```python
from build123d import *

# Parameters (mm, degrees)
SKETCH_1_W          = 30
SKETCH_1_H          = 20
EXTRUDE_1_DEPTH     = 30
SKETCH_3_W          = 25
SKETCH_3_H          = 16.07
EXTRUDE_2_DEPTH     = 10
SKETCH_7_W          = 8
SKETCH_7_H          = 10.5
CUT_EXTRUDE_1_DEPTH = 45.426074479
SKETCH_9_W          = 17
SKETCH_9_H          = 26
CUT_EXTRUDE_2_DEPTH = 25
SKETCH_11_R         = 1.4
EXTRUDE_3_DEPTH     = 4
SKETCH_12_R         = 1.4
EXTRUDE_4_DEPTH     = 4


with BuildPart() as part:
    # 草图1 → 凸台-拉伸1 (new body)
    with BuildSketch(Plane(origin=(0, 0, 0), x_dir=(1, 0, 0), z_dir=(0, 1, 0))):
        with Locations((-0.371492922, 2.183544304)):
            Rectangle(SKETCH_1_W, SKETCH_1_H)
    extrude(amount=EXTRUDE_1_DEPTH)

    # 草图3 → 凸台-拉伸2 (add)
    with BuildSketch(Plane.XY.offset(7.816455696)):
        with Locations((-0.371492922, 15)):
            Rectangle(SKETCH_3_W, SKETCH_3_H)
    extrude(amount=EXTRUDE_2_DEPTH)

    # 草图7 → 切除-拉伸1 (cut, through all)
    with BuildSketch(Plane.ZY.offset(12.871492922)):
        with Locations((13.816455696, 15)):
            Rectangle(SKETCH_7_W, SKETCH_7_H)
    extrude(amount=-CUT_EXTRUDE_1_DEPTH, mode=Mode.SUBTRACT)

    # 草图9 → 切除-拉伸2 (cut)
    with BuildSketch(Plane.ZY.offset(15.371492922)):
        with Locations((-2.183544304, 15)):
            Rectangle(SKETCH_9_W, SKETCH_9_H)
    extrude(amount=-CUT_EXTRUDE_2_DEPTH, mode=Mode.SUBTRACT)

    # 草图11 → 凸台-拉伸3 (add)
    with BuildSketch(Plane(origin=(14.628507078, 0, 0), x_dir=(0, 0, -1), z_dir=(1, 0, 0))):
        with Locations(Location((-2.116455696, 7, 0), (0, 0, 180))):
            Circle(SKETCH_11_R)
        with Locations(Location((6.483544304, 7, 0), (0, 0, 180))):
            Circle(SKETCH_11_R)
    extrude(amount=EXTRUDE_3_DEPTH)

    # 草图12 → 凸台-拉伸4 (add)
    with BuildSketch(Plane(origin=(0, 0, -12.183544304), x_dir=(-1, 0, 0), z_dir=(0, 0, -1))):
        with Locations(Location((-3.928507078, 7, 0), (0, 0, 180))):
            Circle(SKETCH_12_R)
        with Locations(Location((4.671492922, 7, 0), (0, 0, 180))):
            Circle(SKETCH_12_R)
    extrude(amount=EXTRUDE_4_DEPTH)


solid = part.part
```
Build history of the part. All positions in model axes, mm. A direction names the side the tool comes from. Round coordinates to 2 decimals unless told otherwise and drop trailing zeros. Loops run counter-clockwise (first coordinate to the right, second up) from the corner with the lowest first, then second, coordinate; pieces in that order, holes last.
Item 1: Which spindle directions (+Z, -Z, +X, -X, +Y, -Y) get a long thin tool onto all of the face, cutting with end or side? Do faces 1 (the face through (-12.871, 13, 9)), 2 (the face through (-3, 15, -10.684)), 3 (the face through (-1, 20.25, 14)), 4 (the face through (4.575, 8.242, -14.156)), 5 (the face through (-1, 23.035, 13)). Say none if no direction does.
Item 2: Saw through at B-B (x = 11). List the corners of the cut face in (y, z) (3 decimals).
Item 3: Saw through at D-D (y = 26.25). List the corners of the cut face in (x, z), then the cut area to 3 significant figures.
Item 4: Drill centre lines: line 1 along Z through (x, y) = (5, 17.25); line 2 along Y through (x, z) = (1, 6); line 3 along Y through (x, z) = (8, 13) (3 decimals). Where is each one in solid material? Low to high.
Item 5: Pin check, flat tips, straight feed: P1, Ø3, axis at x = 2.5, y = 14.5, coming from the +Z side; P2, Ø8, axis at y = 12, z = 13, coming from the +X side; P3, Ø8, axis at y = 21.5, z = -6.5, coming from the -X side. Stop position of each tip, or through.
Item 6: Two-plate mould, pull along Z, no slides. Class faces 6 (the face through (16.601, 8.242, 2.762)), 7 (the face through (-5, 7, -16.184)), 8 (the face through (-1, 0, -2)): released by +Z, released by -Z, zero draft, split by the parting line, or undercut.
Item 7: Saw through at C-C (z = -9). List the corners of the cut face in (x, y), then the cut area to 3 significant figures.
Worked answers:
1. face 1: +Z, -X, +Y, -Y
1. face 2: -X
1. face 3: +Z, +X, -X
1. face 4: -Z
1. face 5: +Z, +X, -X, +Y
2. outline: (0, -12.184) - (30, -12.184) - (30, 7.816) - (23.035, 7.816) - (23.035, 17.816) - (20.25, 17.816) - (20.25, 9.816) - (9.75, 9.816) - (9.75, 17.816) - (6.965, 17.816) - (6.965, 7.816) - (0, 7.816) - close
3. outline: (-15.37, -12.18) - (14.63, -12.18) - (14.63, 7.82) - (-15.37, 7.82) - (-15.37, 6.32) - (9.63, 6.32) - (9.63, -10.68) - (-15.37, -10.68) - close
3. area: 175 mm2
4. line 1: z = -12.18 to -10.68, 6.32 to 9.82
4. line 2: y = 0 to 2, 28 to 30
4. line 3: y = 6.965 to 9.75, 20.25 to 23.035
5. P1: stops at z = 9.82
5. P2: stops at x = 12.13
5. P3: stops at x = 9.63
6. face 6: undercut
6. face 7: released by -Z
6. face 8: zero draft
7. outline: (-15.37, 0) - (14.63, 0) - (14.63, 30) - (-15.37, 30) - (-15.37, 28) - (9.63, 28) - (9.63, 2) - (-15.37, 2) - close
7. area: 250 mm2
